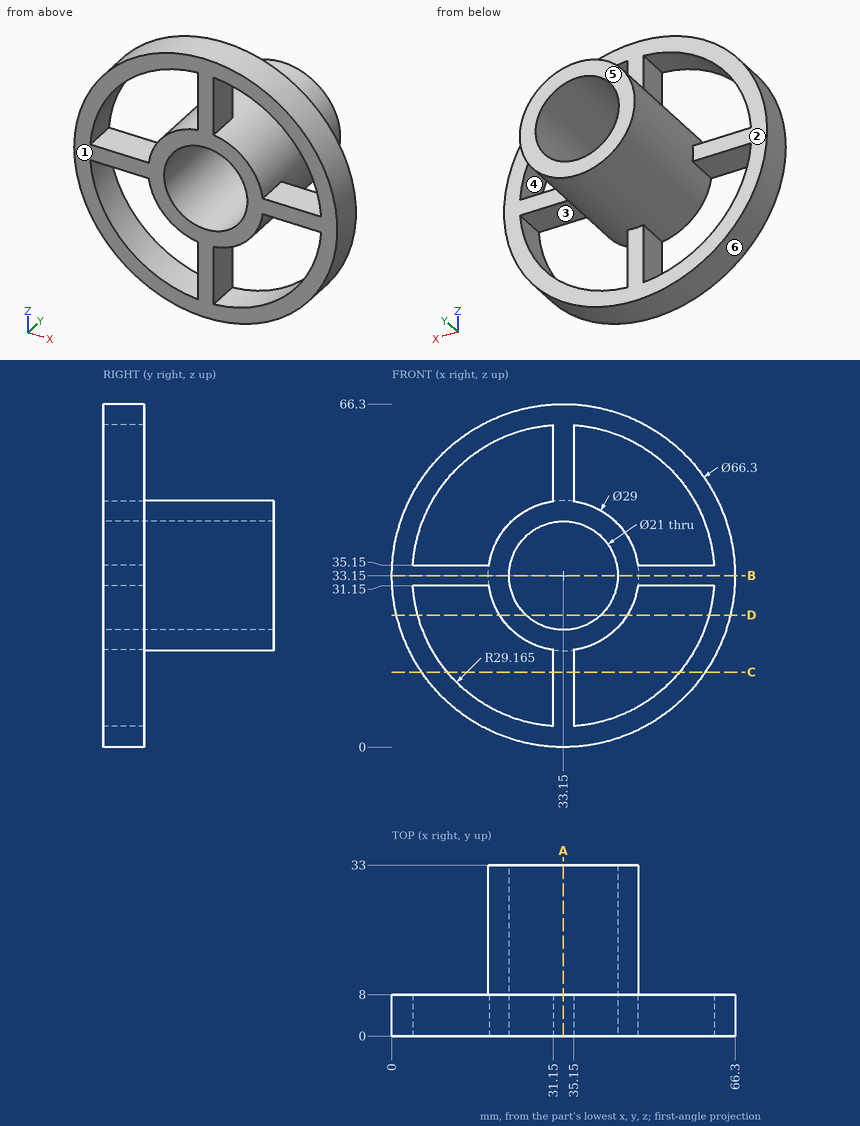
Geometry: see drawing. Coordinates: mm, zero at the bounding-box minimum. A direction names the side the tool comes from. Round coordinates to 2 decimals unless told otherwise and drop trailing zeros. Write each loop counter-clockwise with the first axis right and the second up, starting at its lowest first coordinate (ties: lowest second). Pieces come first, ordered by that corner, then holes. Notation, with made-up numbers: M -30,-16.75 L 25,-16.75 A10 cw 25,-0.75 Z; hole C 67.5,32 d11. An arc over 180 degrees is marked long. Answer in a Markdown table with one row per item. Add a question column.
(1) Reachability of the marked faces 1, 2 and 3 from +Z, -Z, +X, -X, +Y, -Y: full face, straight path, thin tool, end or side. Return the list, or none.
(2) Cut plane C-C, the plane z = 14.5. Return the cut outline in (x, y), then the cut area to 3 significant figures.
(3) Cut plane D-D, the plane z = 25.5. Return the cut outline in (x, y), then the cut area to 3 significant figures.
(4) Ray query, L1, parallel to Z at x = 33, y = 25.5; L2, parallel to Z at x = 31, y = 5.5. Return the intervals inside material, ascending.
(5) Cut plane A-A, the plane x = 33.15. Return the cut outline in (y, z).
(6) Draft query along Z for the marked faces 4, 5 and 6. Return one class per face: pulls with the +Z half, pulls with the -Z half, needs draft (parallel to the pull), parting line crosses it, or undercut.
(7) Contact query for flat-ended pins moving along their axis: pin 1 (2.5 mm diameter, centred on x = 15, y = 4, fed in from +Z); pin 2 (4 mm diameter, centred on x = 8, y = 3, fed in from -Z); pin 3 (6 mm diameter, centred on x = 12.5, z = 33, fed in from +Y); pin 4 (12.5 mm diameter, centred on x = 33.15, z = 33.15, fed in from +Y). Output: stop coordinate, or through.
(8) Cut plane B-B, the plane z = 33.15. Return the cut outline in (x, y), then the cut area to 3 significant figures.
Established:
| question | item | result |
|---|---|---|
| 1 | face 1 | +Z, -Z, +X, -X, -Y |
| 1 | face 2 | +Y |
| 1 | face 3 | +Y, -Y |
| 2 | outline | M 5.74,0 L 10.73,0 L 10.73,8 L 5.74,8 Z; M 31.15,0 L 35.15,0 L 35.15,8 L 31.15,8 Z; M 55.57,0 L 60.56,0 L 60.56,8 L 55.57,8 Z |
| 2 | area | 112 mm² |
| 3 | outline | M 0.89,0 L 5.01,0 L 5.01,8 L 0.89,8 Z; M 20.83,0 L 25.96,0 L 25.96,33 L 20.83,33 Z; M 40.34,0 L 45.47,0 L 45.47,33 L 40.34,33 Z; M 61.29,0 L 65.41,0 L 65.41,8 L 61.29,8 Z |
| 3 | area | 404 mm² |
| 4 | L1 | 18.65 to 22.65, 43.65 to 47.65 |
| 4 | L2 | 0.07 to 4.06, 18.81 to 22.87, 43.43 to 47.49, 62.24 to 66.23 |
| 5 | outline | M 0,0 L 8,0 L 8,18.65 L 33,18.65 L 33,22.65 L 0,22.65 Z; M 0,43.65 L 33,43.65 L 33,47.65 L 8,47.65 L 8,66.3 L 0,66.3 Z |
| 6 | face 4 | undercut |
| 6 | face 5 | needs draft |
| 6 | face 6 | parting line crosses it |
| 7 | pin 1 | z = 61.67 |
| 7 | pin 2 | z = 9.42 |
| 7 | pin 3 | y = 8 |
| 7 | pin 4 | through |
| 8 | outline | M 0,0 L 22.65,0 L 22.65,33 L 18.65,33 L 18.65,8 L 0,8 Z; M 43.65,0 L 66.3,0 L 66.3,8 L 47.65,8 L 47.65,33 L 43.65,33 Z |
| 8 | area | 562 mm² |
